The model under review builds one solid part; all positions refer to its coordinate system, in mm. Round coordinates to 2 decimals unless told otherwise and drop trailing zeros. Write each loop counter-clockwise with the first axis right and the second up, starting at its lowest first coordinate (ties: lowest second). Pieces come first, ordered by that corner, then holes. Notation, with made-up numbers: M 47,28 L 82,28 A14 cw 82,50 Z; hole C 75.25,23 d7. An arc over 180 degrees is marked long. One line per item, written item: value. Start each with the question number.
1) Take a section at A-A, the plane z = -470. Write out the cut boundary in (x, y).
2) Wall thickness on probe 1 along Y at (x, z) = (1.5, 63); probe 2 along X at (y, z) = (3.5, -108); probe 3 along X at (y, z) = (8, 123.5): over which ranges is each line inside the solid? List them lowest first.
3) Take a section at C-C, the plane y = 11. Write out the cut boundary in (x, z).
4) Take a section at B-B, the plane x = -470. Write out the cut boundary in (y, z).
5) Take a section at D-D, the plane z = 0. Write out the cut boundary in (x, y), and give its area (3 significant figures).
6) For P1, Ø8, axis at x = -108, y = 17.5, coming from the +Z side; P2, Ø10, axis at x = -288, y = 8.5, coming from the +Z side; P3, Ø1.5, axis at y = 26, z = -162.5, coming from the +X side, all flat-tipped, find the tip position at first contact; note any pin that passes through.
from build123d import *

# Parameters (mm, degrees)
SKETCH1_R           = 540
BOSS_EXTRUDE1_DEPTH = 30
SKETCH7_R           = 27
BOSS_EXTRUDE2_DEPTH = 5.5
SKETCH10_R          = 26.3
CUT_EXTRUDE1_DEPTH  = 5
SKETCH11_R          = 27
BOSS_EXTRUDE3_DEPTH = 5.5
SKETCH12_R          = 26.3
CUT_EXTRUDE2_DEPTH  = 5
SKETCH13_R          = 26.3
CUT_EXTRUDE3_DEPTH  = 5
SKETCH14_R          = 26.3
CUT_EXTRUDE4_DEPTH  = 5


with BuildPart() as part:
    # Sketch1 → Boss-Extrude1 (new body)
    with BuildSketch(Plane(origin=(0, 0, 0), x_dir=(1, 0, 0), z_dir=(0, 1, 0))):
        with Locations(Location((0, 0, 0), (0, 0, 270))):
            Circle(SKETCH1_R)
    extrude(amount=BOSS_EXTRUDE1_DEPTH)

    # Sketch7 → Boss-Extrude2 (add)
    with BuildSketch(Plane(origin=(0, 30, 0), x_dir=(1, 0, 0), z_dir=(0, 1, 0))):
        with Locations(Location((-470, 0, 0), (0, 0, 270))):
            Circle(SKETCH7_R)
    boss_extrude2 = extrude(amount=BOSS_EXTRUDE2_DEPTH)

    # Sketch10 → Cut-Extrude1 (cut)
    with BuildSketch(Plane(origin=(0, 35.5, 0), x_dir=(1, 0, 0), z_dir=(0, 1, 0))):
        with Locations(Location((-470, 0, 0), (0, 0, 270))):
            Circle(SKETCH10_R)
    extrude(amount=-CUT_EXTRUDE1_DEPTH, mode=Mode.SUBTRACT)

    # Mirror1: Boss-Extrude2 across plane
    add(boss_extrude2.mirror(Plane(origin=(0, 0, 0), x_dir=(0, 0, 1), z_dir=(1, 0, 0))))

    # Sketch11 → Boss-Extrude3 (add)
    with BuildSketch(Plane(origin=(0, 30, 0), x_dir=(1, 0, 0), z_dir=(0, 1, 0))):
        with Locations(Location((0, 470, 0), (0, 0, 270))):
            Circle(SKETCH11_R)
    boss_extrude3 = extrude(amount=BOSS_EXTRUDE3_DEPTH)

    # Sketch12 → Cut-Extrude2 (cut)
    with BuildSketch(Plane(origin=(0, 35.5, 0), x_dir=(1, 0, 0), z_dir=(0, 1, 0))):
        with Locations(Location((0, 469.354248554, 0), (0, 0, 270))):
            Circle(SKETCH12_R)
    extrude(amount=-CUT_EXTRUDE2_DEPTH, mode=Mode.SUBTRACT)

    # Mirror2: Boss-Extrude3 across plane
    add(boss_extrude3.mirror(Plane.XY))

    # Sketch13 → Cut-Extrude3 (cut)
    with BuildSketch(Plane(origin=(0, 35.5, 0), x_dir=(1, 0, 0), z_dir=(0, 1, 0))):
        with Locations(Location((0.231268316, -470.275017284, 0), (0, 0, 270))):
            Circle(SKETCH13_R)
    extrude(amount=-CUT_EXTRUDE3_DEPTH, mode=Mode.SUBTRACT)

    # Sketch14 → Cut-Extrude4 (cut)
    with BuildSketch(Plane(origin=(0, 35.5, 0), x_dir=(1, 0, 0), z_dir=(0, 1, 0))):
        with Locations(Location((470.23112187, -0.273591473, 0), (0, 0, 270))):
            Circle(SKETCH14_R)
    extrude(amount=-CUT_EXTRUDE4_DEPTH, mode=Mode.SUBTRACT)


solid = part.part
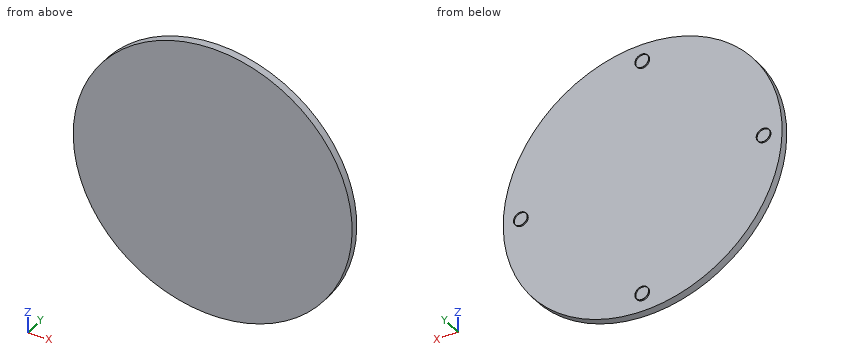
Checked values:
1. outline: M -265.89,0 L 265.89,0 L 265.89,30 L 27,30 L 27,35.5 L 26.29,35.5 L 26.29,30.5 L -26.29,30.5 L -26.29,35.5 L -27,35.5 L -27,30 L -265.89,30 Z
2. probe 1: y = 0 to 30
2. probe 2: x = -529.09 to 529.09
2. probe 3: x = -525.69 to 525.69
3. outline: C 0,0 d1080
4. outline: M 0,-265.89 L 30,-265.89 L 30,-27 L 35.5,-27 L 35.5,-26.3 L 30.5,-26.3 L 30.5,26.3 L 35.5,26.3 L 35.5,27 L 30,27 L 30,265.89 L 0,265.89 Z
5. outline: M -540,0 L 540,0 L 540,30 L 497,30 L 497,35.5 L 496.53,35.5 L 496.53,30.5 L 443.93,30.5 L 443.93,35.5 L 443,35.5 L 443,30 L -443,30 L -443,35.5 L -443.7,35.5 L -443.7,30.5 L -496.3,30.5 L -496.3,35.5 L -497,35.5 L -497,30 L -540,30 Z
5. area: 32,500 mm2
6. P1: stops at z = 529.89
6. P2: stops at z = 459.9
6. P3: stops at x = 515.21
